Geometry: final body of the model. Coordinates: model frame, mm. Face numbers are marked on the shaded views. Give positions to 0.01 mm unless a question says otherwise; leave off trailing zeros. Order: outer loops, then holes, each group sorted by start corner. A loop starts at its lowest first (then second) coordinate and runs counter-clockwise, first axis right, second up. Notation, with made-up numbers: (25, 71.5) - (74, 71.5) arc R29 ccw to (74, 96.5) - close; hole circle Ø5 at (29.25, 77). An arc over 180 degrees is marked (long way). Write item = value, one per line. Start each with the question number.
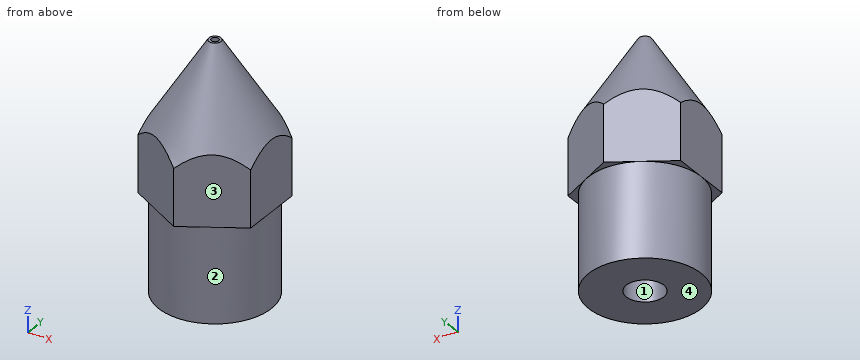
from build123d import *

# Parameters (mm, degrees)
SKETCH4_OUTSIDE_W  = 12.184
SKETCH4_OUTSIDE_H  = 12.184
CUT_EXTRUDE5_DEPTH = 14


with BuildPart() as part:
    # Sketch1 → Revolve2 (revolve)
    with BuildSketch(Plane(origin=(0, 0, 0), x_dir=(0, 0, -1), z_dir=(1, 0, 0))):
        Polygon((0, 0.2), (0, 0.325), (5, 3.464101615), (8, 3.464101615), (8, 3), (13, 3), (13, 1), (3, 1), (0.5, 0.2), align=None)
    revolve(axis=Axis((0, 0, 0), (0, 0, -1)))

    # Sketch4 outside → Cut-Extrude5 (cut, through all)
    with BuildSketch(Plane.XY):
        Rectangle(SKETCH4_OUTSIDE_W, SKETCH4_OUTSIDE_H)
        Polygon((0, 3.464101615), (-3, 1.732050808), (-3, -1.732050808), (0, -3.464101615), (3, -1.732050808), (3, 1.732050808), align=None, mode=Mode.SUBTRACT)
    extrude(amount=-CUT_EXTRUDE5_DEPTH, mode=Mode.SUBTRACT)


solid = part.part
Q1. Section B-B, the plane z = -3.25. Return the cut outline in (x, y), then the cut area to 3 significant figures.
Q2. Contact query for flat-ended pins moving along their axis: pin 1 (2 mm diameter, centred on x = 2, y = 1, fed in from +Z); pin 2 (1.5 mm diameter, centred on x = 1, z = -4.5, fed in from -Y); pin 3 (3 mm diameter, centred on x = 1, z = -8, fed in from -Y); pin 4 (1 mm diameter, centred on x = 1, z = -2, fed in from -Y). Output: stop coordinate, or through.
Q3. Section A-A, the plane z = -11.5. Return the cut outline in (x, y).
Q4. Pull-direction query (Y, two-part tool) for the marked faces 1, 2, 3 and 4; classes: +Y half, -Y half, draft (parallel to the pull), parting line (faces both ways), or undercut.
Q5. Material intervals for line 1 along X through (y, z) = (0, -10.25); line 2 along X through (y, z) = (0, -0.15); line 3 along Z through (x, y) = (2.5, 0), sorted ascending. Write a range as from..to.
The answers:
q1.outline = circle Ø4.73 at (0, 0); hole circle Ø2 at (0, 0)
q1.area = 14.4 mm²
q2.pin_1 = -1.45
q2.pin_2 = -3.29
q2.pin_3 = -3.46
q2.pin_4 = -1.69
q3.outline = circle Ø6 at (0, 0); hole circle Ø2 at (0, 0)
q4.face_1 = undercut
q4.face_2 = parting line
q4.face_3 = -Y half
q4.face_4 = draft
q5.line_1 = -3..-1, 1..3
q5.line_2 = -0.42..-0.2, 0.2..0.42
q5.line_3 = -13..-3.46
